from build123d import *

# Parameters (mm, degrees)
BOSS_EXTRUDE1_DEPTH = 189
SKETCH3_W           = 1.8
SKETCH3_H           = 1
BOSS_EXTRUDE2_DEPTH = 189
FILLET1_START       = -4
FILLET1_DEPTH       = 9


with BuildPart() as part:
    # Sketch1 → Boss-Extrude1 (new body)
    with BuildSketch(Plane.XY):
        Polygon((-2.657407407, 0), (3.742592593, 0), (3.742592593, 3), (1.742592593, 3), (1.742592593, 1.476851852), (-0.657407407, 1.476851852), (-0.657407407, 3), (-2.657407407, 3), align=None)
    extrude(amount=BOSS_EXTRUDE1_DEPTH)

    # Sketch3 → Boss-Extrude2 (add)
    with BuildSketch(Plane.XY.offset(189)):
        with Locations((0.542592593, -0.5)):
            Rectangle(SKETCH3_W, SKETCH3_H)
    extrude(amount=-BOSS_EXTRUDE2_DEPTH)

    # Fillet1: read off the stored shape, not the designer's step
    # Fillet1 outline → Fillet1 (cut)
    with BuildSketch(Plane.YZ.offset(FILLET1_START)):
        with BuildLine():
            Line((-1, 0), (3, 0))
            Line((3, 0), (3, 4.898979486))
            ThreePointArc((3, 4.898979486), (1.872983346, 1.736701826), (-1, 0))
        make_face()
        with BuildLine():
            ThreePointArc((-1, 189), (1.872983346, 187.263298174), (3, 184.101020514))
            Line((3, 184.101020514), (3, 189))
            Line((3, 189), (-1, 189))
        make_face()
    extrude(amount=FILLET1_DEPTH, mode=Mode.SUBTRACT)


solid = part.part
Part model, mm, in its own coordinate system. Give positions to 0.01 mm unless a question says otherwise; leave off trailing zeros. Order: outer loops, then holes, each group sorted by start corner. A loop starts at its lowest first (then second) coordinate and runs counter-clockwise, first axis right, second up. Notation, with made-up numbers: (-35.5, 76.25) - (0.5, 76.25) arc R23 cw to (0.5, 87.25) - close; hole circle Ø9 at (67.5, 46.5). An arc over 180 degrees is marked (long way). Use a Markdown table: item, result.
1) Probe L1, parallel to X at y = 2.35, z = 79; L2, parallel to Y at x = 2.5, z = 70; L3, parallel to X at y = -0.2, z = 57. List the from-to ranges inside material, lowest first. Write a range as from..to.
Checked values:
| item | result |
|---|---|
| L1 | -2.66..-0.66, 1.74..3.74 |
| L2 | 0..3 |
| L3 | -0.36..1.44 |
2) Flat gauge pins, fed straight in: P1, Ø1, axis at x = 1.5, y = 1.5, coming from the -Z side; P2, Ø1.2, axis at x = 0.5, z = 132, coming from the +Y side; P3, Ø0.5, axis at y = -0.5, z = 80, coming from the -X side. Where does each tip first touch, or does it go through?
Checked values:
| item | result |
|---|---|
| P1 | z = 0.9 |
| P2 | y = 1.48 |
| P3 | x = -0.36 |
3) Saw through at B-B on x = 2.75. List the corners of the cut face in (y, z), plus the area to 3 significant figures.
Checked values:
| item | result |
|---|---|
| outline | (0, 0.32) arc R5 ccw to (3, 4.9) - (3, 184.1) arc R5 ccw to (0, 188.68) - close |
| area | 557 mm² |
4) Saw through at A-A on z = 12.5. List the corners of the cut face in (x, y).
Checked values:
| item | result |
|---|---|
| outline | (-2.66, 0) - (-0.36, 0) - (-0.36, -1) - (1.44, -1) - (1.44, 0) - (3.74, 0) - (3.74, 3) - (1.74, 3) - (1.74, 1.48) - (-0.66, 1.48) - (-0.66, 3) - (-2.66, 3) - close |
